For this review, take the finished solid that the model builds, in its own axes (mm). Face numbers are marked on the shaded views. A direction names the side the tool comes from. Give positions to 0.01 mm unless a question says otherwise; leave off trailing zeros. Order: outer loops, then holes, each group sorted by start corner. A loop starts at its lowest first (then second) coordinate and runs counter-clockwise, first axis right, second up. Notation, with made-up numbers: (-23, 38) - (35, 38) arc R23 cw to (35, 58) - close; hole circle Ø6 at (76.5, 69.5). An arc over 180 degrees is marked (long way). Use a Markdown table: item, result. Add a question column.
1) We need section A-A on z = 12.7. Write out the cut boundary in (x, y).
2) Clearance check with flat-ended pins moving along their axes: P1, Ø14.5, axis at x = 25.4, y = -12.7, coming from the -Z side; P2, Ø12.5, axis at y = -16, z = 128.5, coming from the +X side. State where each tip first meets the part, or that it passes through.
3) Wall thickness on L1, parallel to Z at x = 1.15, y = -12.7 (3 decimals); L2, parallel to Y at x = 25.4, z = 186.15; L3, parallel to X at y = -20.75, z = 36.5: over which ranges is each line inside the solid? List them lowest first.
4) We need section B-B on y = -12.7. Give the number of separate pieces and of enclosed holes in the cut face, then the cut area to 3 significant figures.
5) We need section D-D on x = 13.5. Write out the cut boundary in (y, z) (1 decimal), then the cut area to 3 significant figures.
6) Machinability: for the marked faces 1 and 2, which of the approach directions +Z, -Z, +X, -X, +Y, -Y give a long, thin tool a straight path to every point of the face, cutting with its end or side? Answer none if there is none.
```python
from build123d import *

# Parameters (mm, degrees)
F1_DEPTH = 25.4
F3_D     = 12.7
F5_D     = 12.7


with BuildPart() as f1:
    # F0 (on Front) → F1 (new body)
    with BuildSketch(Plane.XZ):
        Polygon((0, 187.325), (0, 0), (4.7625, 0), (4.7625, 182.5625), (38.1, 182.5625), (38.1, 187.325), align=None)
    extrude(amount=F1_DEPTH)

    # F3 (through all)
    with Locations(Plane.YZ.offset(4.7625)):
        with Locations((-12.7, 127), (-12.7, 12.7)):
            Hole(F3_D / 2)

    # F5 (through all)
    with Locations(Plane(origin=(0, 0, 182.5625), x_dir=(1, 0, 0), z_dir=(0, 0, -1))):
        with Locations((25.4, 12.7)):
            Hole(F5_D / 2)


solid = f1.part
```
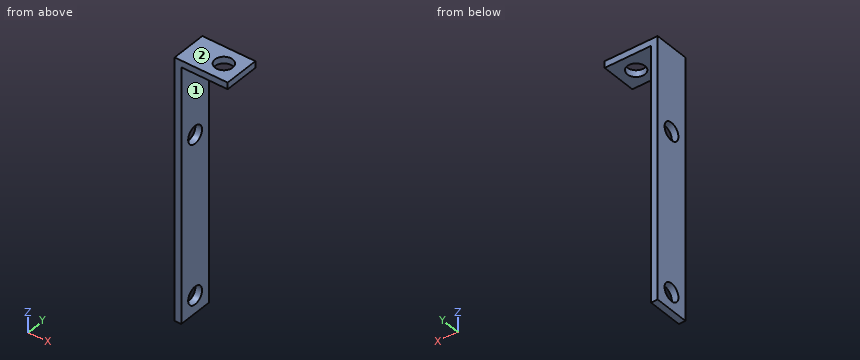
Checked values:
| question | item | result |
|---|---|---|
| 1 | outline | (0, -25.4) - (4.76, -25.4) - (4.76, -19.05) - (0, -19.05) - close; (0, -6.35) - (4.76, -6.35) - (4.76, 0) - (0, 0) - close |
| 2 | P1 | z = 182.56 |
| 2 | P2 | x = 4.76 |
| 3 | L1 | 0 to 6.35, 19.05 to 120.65, 133.35 to 187.325 |
| 3 | L2 | -25.4 to -19.05, -6.35 to 0 |
| 3 | L3 | 0 to 4.76 |
| 4 | separate pieces | 4 |
| 4 | enclosed holes | 0 |
| 4 | area | 869 mm² |
| 5 | outline | (-25.4, 182.6) - (0, 182.6) - (0, 187.3) - (-25.4, 187.3) - close |
| 5 | area | 121 mm² |
| 6 | face 1 | -Z, +X, +Y, -Y |
| 6 | face 2 | +Z, +X, -X, +Y, -Y |
